Verification items for the finished model (mm, model axes). Face numbers are marked on the shaded views. A direction names the side the tool comes from. Give positions to 0.01 mm unless a question says otherwise; leave off trailing zeros. Order: outer loops, then holes, each group sorted by start corner. A loop starts at its lowest first (then second) coordinate and runs counter-clockwise, first axis right, second up. Notation, with made-up numbers: (-1, 19.5) - (51, 19.5) arc R29 cw to (51, 50.5) - close; hole circle Ø4 at (45.5, 81). An arc over 180 degrees is marked (long way). Answer as a JSON object with one key per item and string values. Group by question number.
(1) Section check C-C (y = -5.75). Record the boundary of the cut face in (x, z).
(2) Access from +Z, -Z, +X, -X, +Y, -Y to the whole of each face (thin tool, end or side, straight path). Record for the marked faces 1 and 2.
(3) Section check A-A (x = -1.75). Record the boundary of the cut face in (y, z), then the cut area to 3 significant figures.
(4) Section check B-B (z = 8). Record the boundary of the cut face in (x, y), then the cut area to 3 significant figures.
(5) Thickness scan on line 1 (Z direction, x = -5.75, y = 0); line 2 (Z direction, x = -1, y = -1.25). Record the ranges inside material, lowest first.
(6) Section check D-D (x = 2.5). Record the boundary of the cut face in (y, z).
(7) Mould release check, pull along Z, two halves, no side actions. Record for the marked faces 3, 4 and 5: +Z half, -Z half, draft (parallel to the pull), parting line (faces both ways), or undercut.
(8) Depth check by flat-ended pin: pin 1 Ø3.5 at (y, z) = (-1.5, -1) entering from -X; pin 2 Ø2 at (y, z) = (-3, 2.5) entering from +X; pin 3 Ø0.6 at (x, z) = (-1, 0) entering from +Y; pin 4 Ø1 at (x, y) = (-1, 0) entering from +Z. Enter the tip coordinate at first touch or a pass-through.
```python
from build123d import *

# Parameters (mm, degrees)
SKETCH1_R             = 10
BOSS_EXTRUDE1_DEPTH   = 1
SKETCH3_W             = 6
SKETCH3_H             = 6
BOSS_EXTRUDE2_DEPTH   = 2
SKETCH4_R             = 3
BOSS_EXTRUDE3_DEPTH   = 7
M5_TAPPED_HOLE1_D     = 4.2
M5_TAPPED_HOLE1_DEPTH = 7
M5_TAPPED_HOLE1_TIP   = 1.2618073


with BuildPart() as part:
    # Sketch1 → Boss-Extrude1 (new body)
    with BuildSketch(Plane(origin=(0, 0, 0), x_dir=(0, 0, -1), z_dir=(1, 0, 0))):
        Circle(SKETCH1_R)
    extrude(amount=BOSS_EXTRUDE1_DEPTH)

    # Sketch2 → Revolve1 (revolve)
    with BuildSketch(Plane(origin=(0, 0, 0), x_dir=(1, 0, 0), z_dir=(0, 1, 0))):
        with BuildLine():
            Line((1, 0), (4, 0))
            ThreePointArc((4, 0), (3.233844182, 5.220153254), (1, 10))
            Line((1, 10), (1, 0))
        make_face()
    revolve(axis=Axis((1, 0, 0), (1, 0, 0)))

    # Sketch3 → Boss-Extrude2 (add)
    with BuildSketch(Plane.ZY):
        Rectangle(SKETCH3_W, SKETCH3_H)
    extrude(amount=BOSS_EXTRUDE2_DEPTH)

    # Sketch4 → Boss-Extrude3 (add)
    with BuildSketch(Plane.ZY.offset(2)):
        Circle(SKETCH4_R)
    extrude(amount=BOSS_EXTRUDE3_DEPTH)

    # M5 Tapped Hole1
    with Locations(Plane.ZY.offset(9)):
        with Locations((0, 0)):
            Hole(M5_TAPPED_HOLE1_D / 2, depth=M5_TAPPED_HOLE1_DEPTH)
            with Locations((0, 0, -(M5_TAPPED_HOLE1_DEPTH + M5_TAPPED_HOLE1_TIP / 2))):  # 118° drill point
                Cone(0, M5_TAPPED_HOLE1_D / 2, M5_TAPPED_HOLE1_TIP, mode=Mode.SUBTRACT)


solid = part.part
```
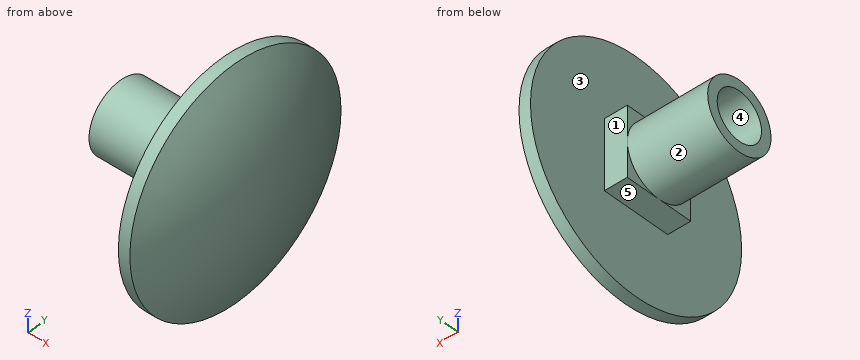
Solutions:
{
 "1": {"outline": "(0, -8.18) - (1, -8.18) arc R17.23 ccw to (1, 8.18) - (0, 8.18) - close"},
 "2": {"face 1": "+Z, -Z, -X, +Y", "face 2": "-X"},
 "3": {"outline": "(-3, -3) - (3, -3) - (3, 3) - (-3, 3) - close; hole circle Ø3.37 at (0, 0)", "area": "27.1 mm2"},
 "4": {"outline": "(0, -6) - (1, -6) arc R16.31 ccw to (1, 6) - (0, 6) - close", "area": "21.2 mm2"},
 "5": {"line 1": "z = -3 to -2.1, 2.1 to 3", "line 2": "z = -3 to 3"},
 "6": {"outline": "circle Ø14.46 at (0, 0)"},
 "7": {"face 3": "draft", "face 4": "undercut", "face 5": "-Z half"},
 "8": {"pin 1": "stops at x = -9", "pin 2": "stops at x = 3.77", "pin 3": "stops at y = 3", "pin 4": "stops at z = 3"}
}
